Verification items for the finished model (mm, model axes). A direction names the side the tool comes from. Give positions to 0.01 mm unless a question says otherwise; leave off trailing zeros. Loops run counter-clockwise (first coordinate to the right, second up) from the corner with the lowest first, then second, coordinate; pieces in that order, holes last. Notation, with made-up numbers: (51, 20.5) -> (96, 20.5) arc R29 ccw to (96, 55.5) -> close; hole circle Ø5 at (77.25, 70). An arc over 180 degrees is marked (long way). Answer in a Markdown table with one row per item. Add a question column.
Q1. Section check A-A on x = 16.25. Enter the section's corners in (y, z).
Q2. Set-up check for faces 1 (the face through (12, 44, 12.8)), 2 (the face through (11.5, 6, 10)), 3 (the face through (18, 15, 8)): record each of +Z, -Z, +X, -X, +Y, -Y from which the full face is reachable in a straight line by a thin tool's end or side.
Q3. Material ranges on probe 1 along Y at (x, z) = (21.7, 6.4); probe 2 along X at (y, z) = (6, 4.5); probe 3 along Y at (x, z) = (14.75, 6.5), recorded low to high.
Q4. Section check C-C on z = 11. Enter the section's corners in (x, y).
Q5. Release check for a two-part mould opening along X. For faces 4 (the face through (18.33, 3.233, 9.666)), 5 (the face through (12.5, 3, 10)), 6 (the face through (24, 25, 11)) record: pulls with the +X half, pulls with the -X half, needs draft (parallel to the pull), parting line crosses it, or undercut.
Q6. Section check B-B on y = 29. Enter the section's corners in (x, z), and give its area (3 significant figures).
Q7. Gauge pin test, flat ends, axial feed: P1, Ø4, axis at y = 4.51, z = 8, coming from the -X side; P2, Ø6.5, axis at x = 9.5, z = 7.5, coming from the +Y side; P3, Ø6.5, axis at x = 9.5, y = 46.5, coming from the -Z side. Record the tip position at first contact, or that the pin passes through.
Q8. Section check D-D on y = 43.9. Enter the section's corners in (x, z), and give its area (3 significant figures).
```python
from build123d import *

# Parameters (mm, degrees)
ESQUISSE1_R             = 6
BOSS_EXTRU_1_DEPTH      = 16
ENL_V_START             = -16
ENL_V_MAT_EXTRU_1_DEPTH = 16
ESQUISSE4_R             = 2.1
ENL_V_MAT_EXTRU_2_DEPTH = 25
ESQUISSE6_W             = 12.8
ESQUISSE6_H             = 12.8
ENL_V_MAT_EXTRU_3_DEPTH = 15
ESQUISSE7_R             = 3
ENL_V_MAT_EXTRU_5_DEPTH = 25
CONG_1_R                = 0.5


with BuildPart() as part:
    # Esquisse1 → Boss.-Extru.1 (new body)
    with BuildSketch(Plane.XY):
        Polygon((0, 0), (24, 0), (24, 24), (24, 51), (0, 51), (0, 30), align=None)
        with Locations((12, 15)):
            Circle(ESQUISSE1_R, mode=Mode.SUBTRACT)
    extrude(amount=BOSS_EXTRU_1_DEPTH)

    # Esquisse2 → Enlèv. mat.-Extru.1 (cut)
    with BuildSketch(Plane(origin=(0, 0, 0), x_dir=(-1, 0, 0), z_dir=(0, 0, -1)).offset(ENL_V_START)):
        with BuildLine():
            Line((-11.5, 31), (-11.5, -14))
            ThreePointArc((-11.5, -14), (-12, -14.5), (-12.5, -14))
            Line((-12.5, -14), (-12.5, 31))
            ThreePointArc((-12.5, 31), (-12, 31.5), (-11.5, 31))
        make_face()
    extrude(amount=ENL_V_MAT_EXTRU_1_DEPTH, mode=Mode.SUBTRACT)

    # Esquisse4 → Enlèv. mat.-Extru.2 (cut, through all)
    with BuildSketch(Plane(origin=(24, 0, 0), x_dir=(0, 0, -1), z_dir=(1, 0, 0))):
        with Locations((-8, 25.989565186)):
            Circle(ESQUISSE4_R)
        with Locations((-8, 4.510434814)):
            Circle(ESQUISSE4_R)
    extrude(amount=-ENL_V_MAT_EXTRU_2_DEPTH, mode=Mode.SUBTRACT)

    # Esquisse6 → Enlèv. mat.-Extru.3 (cut)
    with BuildSketch(Plane(origin=(0, 51, 0), x_dir=(1, 0, 0), z_dir=(0, 1, 0))):
        with Locations((12, -6.4)):
            Rectangle(ESQUISSE6_W, ESQUISSE6_H)
    extrude(amount=-ENL_V_MAT_EXTRU_3_DEPTH, mode=Mode.SUBTRACT)

    # Esquisse7 → Enlèv. mat.-Extru.5 (cut, through all)
    with BuildSketch(Plane(origin=(24, 0, 0), x_dir=(0, 0, -1), z_dir=(1, 0, 0))):
        with Locations((-6.4, 43.9)):
            Circle(ESQUISSE7_R)
    extrude(amount=-ENL_V_MAT_EXTRU_5_DEPTH, mode=Mode.SUBTRACT)

    # Congé1
    cong_1_edges = [part.edges().sort_by_distance(p)[0] for p in [
        (24, 25.5, 16),
        (0, 51, 8),
        (24, 51, 8),
        (24, 0, 8),
        (0, 0, 8),
        (12, 51, 16),
        (18.25, 0, 0),
        (18.25, 0, 16),
        (0, 25.5, 16),
        (0, 25.5, 0),
        (24, 25.5, 0),
        (5.75, 0, 16),
        (5.75, 0, 0),
    ]]
    fillet(cong_1_edges, radius=CONG_1_R)


solid = part.part
```
Taken from the geometry:
| question | item | result |
|---|---|---|
| 1 | outline | (0, 0.5) arc R0.5 ccw to (0.5, 0) -> (10.76, 0) -> (10.76, 16) -> (0.5, 16) arc R0.5 ccw to (0, 15.5) -> close; (19.24, 0) -> (36, 0) -> (36, 12.8) -> (51, 12.8) -> (51, 15.5) arc R0.5 ccw to (50.5, 16) -> (19.24, 16) -> close; hole circle Ø4.2 at (4.51, 8); hole circle Ø4.2 at (25.99, 8) |
| 2 | face 1 | -Z, +Y |
| 2 | face 2 | +Z, -Z, -Y |
| 2 | face 3 | +Z, -Z |
| 3 | probe 1 | y = 0 to 3.15, 5.87 to 24.63, 27.35 to 40.9, 46.9 to 51 |
| 3 | probe 2 | x = 0 to 11.5, 12.5 to 24 |
| 3 | probe 3 | y = 0 to 3.04, 5.98 to 9.67, 20.33 to 24.52, 27.46 to 36 |
| 4 | outline | (0, 0.5) arc R0.5 ccw to (0.5, 0) -> (11.5, 0) -> (11.5, 9.02) arc R6 cw to (11.5, 20.98) -> (11.5, 31) arc R0.5 cw to (12.5, 31) -> (12.5, 20.98) arc R6 cw to (12.5, 9.02) -> (12.5, 0) -> (23.5, 0) arc R0.5 ccw to (24, 0.5) -> (24, 50.5) arc R0.5 ccw to (23.5, 51) -> (18.4, 51) -> (18.4, 36) -> (5.6, 36) -> (5.6, 51) -> (0.5, 51) arc R0.5 ccw to (0, 50.5) -> close |
| 5 | face 4 | needs draft |
| 5 | face 5 | undercut |
| 5 | face 6 | pulls with the +X half |
| 6 | outline | (0, 0.5) arc R0.5 ccw to (0.5, 0) -> (11.5, 0) -> (11.5, 16) -> (0.5, 16) arc R0.5 ccw to (0, 15.5) -> close; (12.5, 0) -> (23.5, 0) arc R0.5 ccw to (24, 0.5) -> (24, 15.5) arc R0.5 ccw to (23.5, 16) -> (12.5, 16) -> close |
| 6 | area | 368 mm² |
| 7 | P1 | passes through |
| 7 | P2 | stops at y = 36 |
| 7 | P3 | stops at z = 12.8 |
| 8 | outline | (0, 0.5) arc R0.5 ccw to (0.5, 0) -> (5.6, 0) -> (5.6, 3.4) -> (0, 3.4) -> close; (0, 9.4) -> (5.6, 9.4) -> (5.6, 12.8) -> (18.4, 12.8) -> (18.4, 9.4) -> (24, 9.4) -> (24, 15.5) arc R0.5 ccw to (23.5, 16) -> (0.5, 16) arc R0.5 ccw to (0, 15.5) -> close; (18.4, 0) -> (23.5, 0) arc R0.5 ccw to (24, 0.5) -> (24, 3.4) -> (18.4, 3.4) -> close |
| 8 | area | 153 mm² |
